Model file for the job. Use its own axes, mm. Face numbers are marked on the shaded views. A direction names the side the tool comes from. Coordinates: 2 decimals unless noted, no trailing zeros. Write each loop counter-clockwise with the first axis right and the second up, starting at its lowest first coordinate (ties: lowest second). Pieces come first, ordered by that corner, then holes. Notation, with made-up numbers: (68, 62) - (96, 62) arc R22 ccw to (96, 69) - close; hole circle Ø9 at (53, -2.75). An arc over 180 degrees is marked (long way). Put each result on its own line as item: value. Start each with the question number.
1. Saw through at C-C, the plane z = -6.5. Write the cut outline in (x, y).
2. Which spindle directions (+Z, -Z, +X, -X, +Y, -Y) get a long thin tool onto all of the face, cutting with end or side? Do the marked faces 1 and 2. Say none if no direction does.
3. Drill centre lines: L1, parallel to Y at x = 42.35, z = -4.15; L2, parallel to X at y = -20.75, z = -11.5; L3, parallel to Y at x = 0.6, z = -11.65. Where is each one in solid material? Low to high. Write a range as from..to.
4. Drop flat-ended pins along their axis: P1, Ø4, axis at x = 4.5, z = -6, coming from the -Y side; P2, Ø1.2, axis at y = -10.9, z = -18.65, coming from the -X side; P3, Ø1.8, axis at y = -18.45, z = -4.15, coming from the +X side. Give the stop position or say it passes through.
5. Saw through at D-D, the plane y = 2.5. Write the cut outline in (x, z).
6. Saw through at B-B, the plane y = -2. Write the cut outline in (x, z).
7. Saw through at A-A, the plane x = 21.5. Write the cut outline in (y, z).
```python
from build123d import *

# Parameters (mm, degrees)
SKETCH1_W                   = 43
SKETCH1_H                   = 23.3
MOUNTPLATE_DEPTH            = 4.6
SKETCH3_R                   = 4.5
AXLEHOLE_MOUNT_DEPTH        = 4.6
SKETCH2_R                   = 1
MOUNTHOLES_DEPTH            = 4.6
SKETCH4_W                   = 1.1
SKETCH4_H                   = 23.3
SERVOLEGS_DEPTH             = 22.4
CENTERHOLES_REACH           = 55.793
SKETCH5_R                   = 4.5
SKETCH6_R                   = 1
ROTORSIDE_MOUNTHOLES_DEPTH  = 1.1
FILLET1_R                   = 11.5
FILLET2_R                   = 11.5
SKETCH7_R                   = 1
SLIDERSIDE_MOUNTHOLES_DEPTH = 1.1


with BuildPart() as part:
    # Sketch1 → MountPlate (new body)
    with BuildSketch(Plane(origin=(0, 0, 0), x_dir=(1, 0, 0), z_dir=(0, 1, 0))):
        with Locations((21.5, 11.65)):
            Rectangle(SKETCH1_W, SKETCH1_H)
    extrude(amount=MOUNTPLATE_DEPTH)

    # Sketch3 → AxleHole-Mount (cut)
    with BuildSketch(Plane(origin=(0, 4.6, 0), x_dir=(1, 0, 0), z_dir=(0, 1, 0))):
        with Locations(Location((21.5, 11.65, 0), (0, 0, 270))):
            Circle(SKETCH3_R)
    extrude(amount=-AXLEHOLE_MOUNT_DEPTH, mode=Mode.SUBTRACT)

    # Sketch2 → MountHoles (cut)
    with BuildSketch(Plane(origin=(0, 4.6, 0), x_dir=(1, 0, 0), z_dir=(0, 1, 0))):
        with Locations(Location((6.59, 11.65, 0), (0, 0, 270))):
            Circle(SKETCH2_R)
        with Locations(Location((16.550252532, 6.700252532, 0), (0, 0, 270))):
            Circle(SKETCH2_R)
        with Locations(Location((36.41, 11.65, 0), (0, 0, 270))):
            Circle(SKETCH2_R)
        with Locations(Location((16.550252532, 16.599747468, 0), (0, 0, 270))):
            Circle(SKETCH2_R)
        with Locations(Location((26.449747468, 16.599747468, 0), (0, 0, 270))):
            Circle(SKETCH2_R)
        with Locations(Location((26.449747468, 6.700252532, 0), (0, 0, 270))):
            Circle(SKETCH2_R)
    extrude(amount=-MOUNTHOLES_DEPTH, mode=Mode.SUBTRACT)

    # Sketch4 → ServoLegs (add)
    with BuildSketch(Plane.XZ):
        with Locations((42.45, -11.65)):
            Rectangle(SKETCH4_W, SKETCH4_H)
        with Locations((0.55, -11.65)):
            Rectangle(SKETCH4_W, SKETCH4_H)
    extrude(amount=SERVOLEGS_DEPTH)

    # CenterHoles: up to this face of the body (flat: up to its plane)
    centerholes_end = Plane(part.part.faces().sort_by_distance((43, -8.9, -11.65))[0])
    # Sketch5 → CenterHoles (cut, up to the picked face)
    with BuildSketch(Plane.ZY, mode=Mode.PRIVATE) as centerholes_sk1:
        with Locations((-11.65, -10.9)):
            Circle(SKETCH5_R)
    centerholes_tool1 = split(extrude(centerholes_sk1.sketch, amount=-CENTERHOLES_REACH, mode=Mode.PRIVATE), bisect_by=centerholes_end, keep=Keep.BOTH, mode=Mode.PRIVATE)
    add(centerholes_tool1.solids().sort_by(Axis((0, -10.9, -11.65), (1, 0, 0)))[0], mode=Mode.SUBTRACT)

    # Sketch6 → RotorSide-MountHoles (cut)
    with BuildSketch(Plane.ZY):
        with Locations((-11.65, -17.9)):
            Circle(SKETCH6_R)
        with Locations((-18.65, -10.9)):
            Circle(SKETCH6_R)
        with Locations((-11.65, -3.9)):
            Circle(SKETCH6_R)
        with Locations((-4.65, -10.9)):
            Circle(SKETCH6_R)
    extrude(amount=-ROTORSIDE_MOUNTHOLES_DEPTH, mode=Mode.SUBTRACT)

    # Fillet1
    fillet1_edges = [part.edges().sort_by_distance(p)[0] for p in [
        (0.55, -22.4, -23.3),
    ]]
    fillet(fillet1_edges, radius=FILLET1_R)

    # Fillet2
    fillet2_edges = [part.edges().sort_by_distance(p)[0] for p in [
        (0.55, -22.4, 0),
    ]]
    fillet(fillet2_edges, radius=FILLET2_R)

    # Sketch7 → SliderSide-MountHoles (cut)
    with BuildSketch(Plane(origin=(43, 0, 0), x_dir=(0, 0, -1), z_dir=(1, 0, 0))):
        with Locations((19.15, -18.45)):
            Circle(SKETCH7_R)
        with Locations((19.15, -3.45)):
            Circle(SKETCH7_R)
        with Locations((4.15, -3.45)):
            Circle(SKETCH7_R)
        with Locations((4.15, -18.45)):
            Circle(SKETCH7_R)
    extrude(amount=-SLIDERSIDE_MOUNTHOLES_DEPTH, mode=Mode.SUBTRACT)


solid = part.part
```
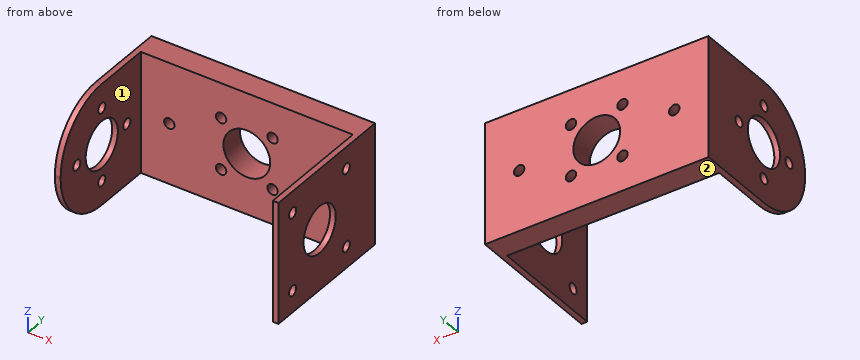
Final values:
1. outline: (0, -21.26) - (1.1, -21.26) - (1.1, 0) - (15.57, 0) - (15.57, 4.6) - (0, 4.6) - close; (17.53, 0) - (25.47, 0) - (25.47, 4.6) - (17.53, 4.6) - close; (27.43, 0) - (41.9, 0) - (41.9, -22.4) - (43, -22.4) - (43, 4.6) - (27.43, 4.6) - close
2. face 1: +Z, -Z, -Y
2. face 2: -Z, +X, -X, +Y, -Y
3. L1: y = -22.4..-19.45, -17.45..-4.45, -2.45..4.6
3. L2: x = 0..1.1, 41.9..43
3. L3: y = -22.4..-18.9, -16.9..-15.4, -6.4..-4.9, -2.9..4.6
4. P1: stops at y = 0
4. P2: stops at x = 41.9
4. P3: stops at x = 1.1
5. outline: (0, -23.3) - (43, -23.3) - (43, 0) - (0, 0) - close; hole circle Ø2 at (6.59, -11.65); hole circle Ø2 at (16.55, -16.6); hole circle Ø2 at (16.55, -6.7); hole circle Ø9 at (21.5, -11.65); hole circle Ø2 at (26.45, -16.6); hole circle Ø2 at (26.45, -6.7); hole circle Ø2 at (36.41, -11.65)
6. outline: (0, -23.3) - (1.1, -23.3) - (1.1, 0) - (0, 0) - close; (41.9, -23.3) - (43, -23.3) - (43, 0) - (41.9, 0) - close
7. outline: (0, -23.3) - (4.6, -23.3) - (4.6, -16.15) - (0, -16.15) - close; (0, -7.15) - (4.6, -7.15) - (4.6, 0) - (0, 0) - close
